from build123d import *

# Parameters (mm, degrees)
ESQUISSE1_W             = 93
ESQUISSE1_H             = 309
BOSS_EXTRU_1_DEPTH      = 3
PERSAGE_STEPPER_DEPTH   = 4
ESQUISSE3_R             = 2.5
ENL_V_MAT_EXTRU_1_DEPTH = 3
ESQUISSE4_R             = 1.75
ENL_V_MAT_EXTRU_2_DEPTH = 3


with BuildPart() as part:
    # Esquisse1 → Boss.-Extru.1 (new body)
    with BuildSketch(Plane.XY):
        with Locations((46.5, 154.5)):
            Rectangle(ESQUISSE1_W, ESQUISSE1_H)
    extrude(amount=BOSS_EXTRU_1_DEPTH)

    # Esquisse2 → Persage Stepper (cut, through all)
    with BuildSketch(Plane.XY.offset(3)):
        with BuildLine():
            Line((34.5, 277.5), (34.5, 287.5))
            ThreePointArc((34.5, 287.5), (46.5, 299.5), (58.5, 287.5))
            Line((58.5, 287.5), (58.5, 277.5))
            ThreePointArc((58.5, 277.5), (46.5, 265.5), (34.5, 277.5))
        make_face()
        with BuildLine():
            Line((29.5, 293), (29.5, 303))
            ThreePointArc((29.5, 303), (31, 304.5), (32.5, 303))
            Line((32.5, 303), (32.5, 293))
            ThreePointArc((32.5, 293), (31, 291.5), (29.5, 293))
        make_face()
        with BuildLine():
            Line((60.5, 293), (60.5, 303))
            ThreePointArc((60.5, 303), (62, 304.5), (63.5, 303))
            Line((63.5, 303), (63.5, 293))
            ThreePointArc((63.5, 293), (62, 291.5), (60.5, 293))
        make_face()
        with BuildLine():
            Line((60.5, 262), (60.5, 272))
            ThreePointArc((60.5, 272), (62, 273.5), (63.5, 272))
            Line((63.5, 272), (63.5, 262))
            ThreePointArc((63.5, 262), (62, 260.5), (60.5, 262))
        make_face()
        with BuildLine():
            Line((29.5, 262), (29.5, 272))
            ThreePointArc((29.5, 272), (31, 273.5), (32.5, 272))
            Line((32.5, 272), (32.5, 262))
            ThreePointArc((32.5, 262), (31, 260.5), (29.5, 262))
        make_face()
    extrude(amount=-PERSAGE_STEPPER_DEPTH, mode=Mode.SUBTRACT)

    # Esquisse3 → Enlèv. mat.-Extru.1 (cut)
    with BuildSketch(Plane.XY.offset(3)):
        with Locations((46.5, 10)):
            Circle(ESQUISSE3_R)
    extrude(amount=-ENL_V_MAT_EXTRU_1_DEPTH, mode=Mode.SUBTRACT)

    # Esquisse4 → Enlèv. mat.-Extru.2 (cut)
    with BuildSketch(Plane.XY.offset(3)):
        with Locations((10, 12.5)):
            Circle(ESQUISSE4_R)
        with Locations((83, 12.5)):
            Circle(ESQUISSE4_R)
        with Locations((10, 37.5)):
            Circle(ESQUISSE4_R)
        with Locations((83, 37.5)):
            Circle(ESQUISSE4_R)
        with Locations((10, 62.5)):
            Circle(ESQUISSE4_R)
        with Locations((83, 62.5)):
            Circle(ESQUISSE4_R)
        with Locations((10, 87.5)):
            Circle(ESQUISSE4_R)
        with Locations((83, 87.5)):
            Circle(ESQUISSE4_R)
        with Locations((10, 112.5)):
            Circle(ESQUISSE4_R)
        with Locations((83, 112.5)):
            Circle(ESQUISSE4_R)
        with Locations((10, 137.5)):
            Circle(ESQUISSE4_R)
        with Locations((83, 137.5)):
            Circle(ESQUISSE4_R)
        with Locations((10, 162.5)):
            Circle(ESQUISSE4_R)
        with Locations((83, 162.5)):
            Circle(ESQUISSE4_R)
        with Locations((10, 187.5)):
            Circle(ESQUISSE4_R)
        with Locations((83, 187.5)):
            Circle(ESQUISSE4_R)
        with Locations((10, 212.5)):
            Circle(ESQUISSE4_R)
        with Locations((83, 212.5)):
            Circle(ESQUISSE4_R)
        with Locations((10, 237.5)):
            Circle(ESQUISSE4_R)
        with Locations((83, 237.5)):
            Circle(ESQUISSE4_R)
        with Locations((10, 262.5)):
            Circle(ESQUISSE4_R)
        with Locations((83, 262.5)):
            Circle(ESQUISSE4_R)
        with Locations((10, 287.5)):
            Circle(ESQUISSE4_R)
        with Locations((83, 287.5)):
            Circle(ESQUISSE4_R)
    extrude(amount=-ENL_V_MAT_EXTRU_2_DEPTH, mode=Mode.SUBTRACT)


solid = part.part
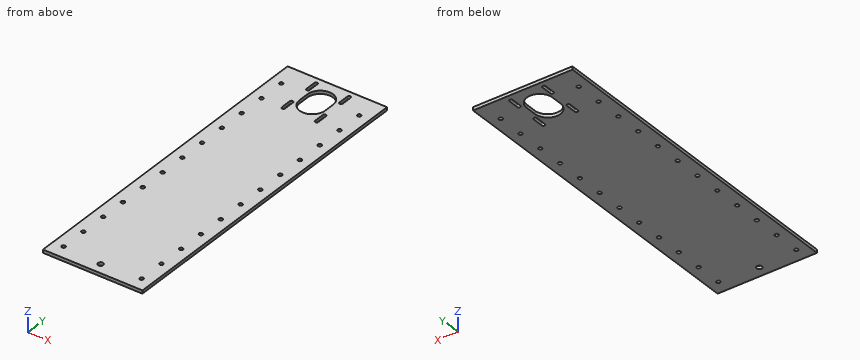
Read the model definition and answer for the solid it produces. Units are mm, in the model's axes. Give positions to 0.01 mm unless a question says otherwise; leave off trailing zeros. Loops run counter-clockwise (first coordinate to the right, second up) from the corner with the lowest first, then second, coordinate; pieces in that order, holes last. Notation, with made-up numbers: (17, -21) -> (45, -21) arc R6 ccw to (45, -11) -> close; hole circle Ø4 at (-23.5, 81). An arc over 180 degrees is marked (long way). Use a Markdown table: item, result.
Q1. Section A-A, the plane x = 54.5 is taken. Determine the outline of the cut face in (y, z), then the cut area to 3 significant figures.
Solved:
| item | result |
|---|---|
| outline | (0, 0) -> (268.56, 0) -> (268.56, 3) -> (0, 3) -> close; (296.44, 0) -> (309, 0) -> (309, 3) -> (296.44, 3) -> close |
| area | 843 mm^2 |
Q2. Find the intervals of material crossed by line 1 along X through (y, z) = (187.5, 1.95); line 2 along X through (y, z) = (262.5, 2.4); line 3 along Y through (x, z) = (62.5, 1.55), in increasing order.
Solved:
| item | result |
|---|---|
| line 1 | x = 0 to 8.25, 11.75 to 81.25, 84.75 to 93 |
| line 2 | x = 0 to 8.25, 11.75 to 29.5, 32.5 to 60.5, 63.5 to 81.25, 84.75 to 93 |
| line 3 | y = 0 to 260.59, 273.41 to 291.59, 304.41 to 309 |
Q3. This flat-tipped pin is pushed along its axis until it touches: pin 1 (2 mm diameter, centred on x = 83, y = 37.5, fed in from -Z). Where does it stop, or does it pass through?
Solved:
| item | result |
|---|---|
| pin 1 | passes through |
